Could you check a few things on this model? Use its own coordinates, in mm. Give positions to 0.01 mm unless a question says otherwise; leave off trailing zeros.
1. Thinking about a two-plate mould opening in Z: for faces 1 (the cylindrical face through (280.5, 4.9, -23.1)), 2 (the flat face through (177, 10, -74)), 3 (the flat face through (177, 5, 0)), 4 (the cylindrical face through (79.6, 4.9, -103.2)), which applies, +Z half, -Z half, draft (parallel to the pull), parting line (faces both ways), or undercut?
2. For P1, Ø5, axis at x = 15, z = -5, coming from the +Y side, with a flat end and sliding along its axis, tell me the tip position at first contact or that it passes through.
3. I need wall thicknesses on line 1 along Z through (x, y) = (167, 6.75); line 2 along X through (y, z) = (7.5, -5); line 3 along X through (y, z) = (7.25, -90.5). Which ranges of each line are inside material? Lowest first, please.
```python
from build123d import *

# Parameters (mm, degrees)
SKETCH1_W           = 360
SKETCH1_H           = 145
SKETCH1_R           = 3
BOSS_EXTRUDE1_DEPTH = 10


with BuildPart() as part:
    # Sketch1 → Boss-Extrude1 (new body)
    with BuildSketch(Plane(origin=(0, 0, 0), x_dir=(1, 0, 0), z_dir=(0, 1, 0))):
        with Locations((180, 72.5)):
            Rectangle(SKETCH1_W, SKETCH1_H)
        with Locations((15, 5)):
            Circle(SKETCH1_R, mode=Mode.SUBTRACT)
        with Locations((10, 53)):
            Circle(SKETCH1_R, mode=Mode.SUBTRACT)
        with Locations((92, 53)):
            Circle(SKETCH1_R, mode=Mode.SUBTRACT)
        with Locations((89.5, 5)):
            Circle(SKETCH1_R, mode=Mode.SUBTRACT)
        with Locations((5, 105)):
            Circle(SKETCH1_R, mode=Mode.SUBTRACT)
        with Locations((70, 105)):
            Circle(SKETCH1_R, mode=Mode.SUBTRACT)
        with Locations((82, 105)):
            Circle(SKETCH1_R, mode=Mode.SUBTRACT)
        with Locations((147, 105)):
            Circle(SKETCH1_R, mode=Mode.SUBTRACT)
        with Locations((356, 60)):
            Circle(SKETCH1_R, mode=Mode.SUBTRACT)
        with Locations((356, 129)):
            Circle(SKETCH1_R, mode=Mode.SUBTRACT)
        with Locations((241, 60)):
            Circle(SKETCH1_R, mode=Mode.SUBTRACT)
        with Locations((283.5, 23)):
            Circle(SKETCH1_R, mode=Mode.SUBTRACT)
        with Locations((167, 91)):
            Circle(SKETCH1_R, mode=Mode.SUBTRACT)
        with Locations((167, 119)):
            Circle(SKETCH1_R, mode=Mode.SUBTRACT)
    extrude(amount=BOSS_EXTRUDE1_DEPTH)


solid = part.part
```
Derived:
1. face 1: undercut
1. face 2: draft
1. face 3: +Z half
1. face 4: undercut
2. P1: passes through
3. line 1: z = -145 to -122, -116 to -94, -88 to 0
3. line 2: x = 0 to 12, 18 to 86.5, 92.5 to 360
3. line 3: x = 0 to 164.04, 169.96 to 360
